The model under review builds one solid part; all positions refer to its coordinate system, in mm. Coordinates: 2 decimals unless noted, no trailing zeros. Write each loop counter-clockwise with the first axis right and the second up, starting at its lowest first coordinate (ties: lowest second). Pieces come first, ordered by that corner, then holes. Notation, with made-up numbers: (-20, 15) - (-4, 15) arc R12 cw to (-4, 37) - close; hole circle Ø4 at (4, 19.25). An arc over 180 degrees is marked (long way). Use one line per item in the form item = value. Start each with the question number.
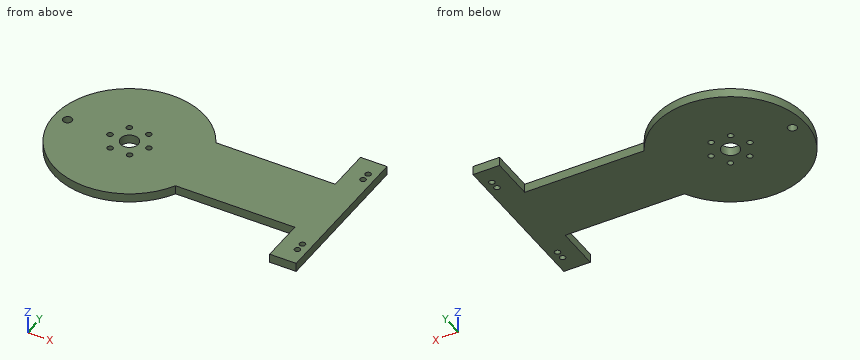
```python
from build123d import *

# Parameters (mm, degrees)
SKETCH_1_R          = 85
EXTRUDE_1_DEPTH     = 10
SKETCH_2_W          = 240
SKETCH_2_H          = 80
EXTRUDE_2_DEPTH     = 10
SKETCH_3_W          = 30
SKETCH_3_H          = 180
EXTRUDE_3_DEPTH     = 10
SKETCH_4_R          = 10
SKETCH_4_R_2        = 3.25
SKETCH_4_R_3        = 5.1
CUT_EXTRUDE_1_DEPTH = 11


with BuildPart() as part:
    # 草图1 → 凸台-拉伸1 (new body)
    with BuildSketch(Plane.XY):
        Circle(SKETCH_1_R)
    extrude(amount=EXTRUDE_1_DEPTH)

    # 草图2 → 凸台-拉伸2 (add)
    with BuildSketch(Plane.XY):
        with Locations((120, 0)):
            Rectangle(SKETCH_2_W, SKETCH_2_H)
    extrude(amount=EXTRUDE_2_DEPTH)

    # 草图3 → 凸台-拉伸3 (add)
    with BuildSketch(Plane.XY):
        with Locations((225, 0)):
            Rectangle(SKETCH_3_W, SKETCH_3_H)
    extrude(amount=EXTRUDE_3_DEPTH)

    # 草图4 → 切除-拉伸1 (cut)
    with BuildSketch(Plane(origin=(0, 0, 0), x_dir=(-1, 0, 0), z_dir=(0, 0, -1))):
        Circle(SKETCH_4_R)
        with Locations((-22, 0)):
            Circle(SKETCH_4_R_2)
        with Locations((-11, 19.052558883)):
            Circle(SKETCH_4_R_2)
        with Locations((11, 19.052558883)):
            Circle(SKETCH_4_R_2)
        with Locations((22, 0)):
            Circle(SKETCH_4_R_2)
        with Locations((11, -19.052558883)):
            Circle(SKETCH_4_R_2)
        with Locations((-11, -19.052558883)):
            Circle(SKETCH_4_R_2)
        with Locations((-230, -70)):
            Circle(SKETCH_4_R_2)
        with Locations((-230, -60)):
            Circle(SKETCH_4_R_2)
        with Locations((-230, 60)):
            Circle(SKETCH_4_R_2)
        with Locations((-230, 70)):
            Circle(SKETCH_4_R_2)
        with Locations((70, 0)):
            Circle(SKETCH_4_R_3)
    extrude(amount=-CUT_EXTRUDE_1_DEPTH, mode=Mode.SUBTRACT)


solid = part.part
```
1. For L1, parallel to Y at x = 230, z = 2.25; L2, parallel to Y at x = 11, z = 8.25; L3, parallel to X at y = -67.5, z = 6.75, list the stretches that pass through material, from the lowest coordinate up.
2. For P1, Ø5, axis at x = 171.5, z = 7.5, coming from the -Y side; P2, Ø5, axis at x = -41, z = 8, coming from the +Y side; P3, Ø2, axis at y = -9, z = 7.5, coming from the -X side, all flat-tipped, find the tip position at first contact; note any pin that passes through.
3. Take a section at B-B (x = 0). State the section outline as (y, z) points.
4. Take a section at A-A (y = 0). State the section outline as (x, z) points, plus the area to 3 significant figures.
5. Take a section at C-C (x = 230). State the section outline as (y, z) points, plus the area to 3 significant figures.
6. Take a section at D-D (y = 60). State the section outline as (x, z) points, plus the area to 3 significant figures.
Returned:
q1.L1 = -90 to -73.25, -66.75 to -63.25, -56.75 to 56.75, 63.25 to 66.75, 73.25 to 90
q1.L2 = -84.29 to -22.3, -15.8 to 15.8, 22.3 to 84.29
q1.L3 = -51.66 to 51.66, 210 to 227.92, 232.08 to 240
q2.P1 = -40
q2.P2 = 75.78
q2.P3 = -84.62
q3.outline = (-85, 0) - (-10, 0) - (-10, 10) - (-85, 10) - close; (10, 0) - (85, 0) - (85, 10) - (10, 10) - close
q4.outline = (-85, 0) - (-75.1, 0) - (-75.1, 10) - (-85, 10) - close; (-64.9, 0) - (-25.25, 0) - (-25.25, 10) - (-64.9, 10) - close; (-18.75, 0) - (-10, 0) - (-10, 10) - (-18.75, 10) - close; (10, 0) - (18.75, 0) - (18.75, 10) - (10, 10) - close; (25.25, 0) - (240, 0) - (240, 10) - (25.25, 10) - close
q4.area = 2,820 mm²
q5.outline = (-90, 0) - (-73.25, 0) - (-73.25, 10) - (-90, 10) - close; (-66.75, 0) - (-63.25, 0) - (-63.25, 10) - (-66.75, 10) - close; (-56.75, 0) - (56.75, 0) - (56.75, 10) - (-56.75, 10) - close; (63.25, 0) - (66.75, 0) - (66.75, 10) - (63.25, 10) - close; (73.25, 0) - (90, 0) - (90, 10) - (73.25, 10) - close
q5.area = 1,540 mm²
q6.outline = (-60.21, 0) - (60.21, 0) - (60.21, 10) - (-60.21, 10) - close; (210, 0) - (226.75, 0) - (226.75, 10) - (210, 10) - close; (233.25, 0) - (240, 0) - (240, 10) - (233.25, 10) - close
q6.area = 1,440 mm²
